```python
from build123d import *

# Parameters (mm, degrees)
F0_W     = 35
F0_H     = 80
F0_H_2   = 120
F2_DEPTH = 1
F4_DEPTH = 2000
F5_DEPTH = 640


# Not quite as in the source:
# - a feature names something its author has since deleted; it is built from what else it names


with BuildPart() as f2:
    # F0 (on Top) → F2 (new body)
    with BuildSketch(Plane.XY):
        Polygon((380, 360), (-380, 360), (-380, -360), (0, -360), (380, -360), align=None)
        with Locations((-260.5, -310)):
            Rectangle(F0_W, F0_H, mode=Mode.SUBTRACT)
        with Locations((260.5, -310)):
            Rectangle(F0_W, F0_H, mode=Mode.SUBTRACT)
        with Locations((-260.5, 250)):
            Rectangle(F0_W, F0_H_2, mode=Mode.SUBTRACT)
        with Locations((260.5, 250)):
            Rectangle(F0_W, F0_H_2, mode=Mode.SUBTRACT)
    extrude(amount=F2_DEPTH)

    # F0 (on Top) → F4 (join)
    with BuildSketch(Plane.XY):
        with Locations((-260.5, 250)):
            Rectangle(F0_W, F0_H_2)
        with Locations((-260.5, -310)):
            Rectangle(F0_W, F0_H)
        with Locations((260.5, -310)):
            Rectangle(F0_W, F0_H)
        with Locations((260.5, 250)):
            Rectangle(F0_W, F0_H_2)
    extrude(amount=F4_DEPTH)

    # F3 (on offset) → F5 (join)
    with BuildSketch(Plane.XZ.offset(350)):
        Polygon((-187.5, 29), (-187.5, 30), (-232.5, 30), (-242.5, 30), (-242.5, 40), (-242.5, 70), (-243.5, 70), (-243.5, 30), (-243.5, 29), align=None)
        Polygon((-242.5, 30), (-232.5, 30), (-242.5, 40), align=None)
        Polygon((242.5, 40), (232.5, 30), (242.5, 30), align=None)
        Polygon((232.5, 30), (187.5, 30), (187.5, 29), (243.5, 29), (243.5, 30), (243.5, 70), (242.5, 70), (242.5, 40), (242.5, 30), align=None)
    extrude(amount=-F5_DEPTH)


solid = f2.part
```
Can you work these out from the model? Positions are in its coordinate system, mm. A direction names the side the tool comes from. Round coordinates to 2 decimals unless told otherwise and drop trailing zeros. Loops run counter-clockwise (first coordinate to the right, second up) from the corner with the lowest first, then second, coordinate; pieces in that order, holes last. Notation, with made-up numbers: (30.25, 78.5) -> (65.25, 78.5) arc R35 ccw to (65.25, 117.5) -> close; hole circle Ø5 at (87, -16). An arc over 180 degrees is marked (long way). Answer in a Markdown table with one row per item.
Item 1: Suppose I cut it at B-B, the plane y = -238. List the corners of the cut face in (x, z) for me, plus the area to 3 significant figures.
Answer block:
| item | result |
|---|---|
| outline | (-380, 0) -> (380, 0) -> (380, 1) -> (-380, 1) -> close; (-243.5, 29) -> (-187.5, 29) -> (-187.5, 30) -> (-232.5, 30) -> (-242.5, 40) -> (-242.5, 70) -> (-243.5, 70) -> close; (187.5, 29) -> (243.5, 29) -> (243.5, 70) -> (242.5, 70) -> (242.5, 40) -> (232.5, 30) -> (187.5, 30) -> close |
| area | 1,050 mm² |
Item 2: Suppose I cut it at A-A, the plane z = 959. List the corners of the cut face in (x, y) for me.
Answer block:
| item | result |
|---|---|
| outline | (-278, -350) -> (-243, -350) -> (-243, -270) -> (-278, -270) -> close; (-278, 190) -> (-243, 190) -> (-243, 310) -> (-278, 310) -> close; (243, -350) -> (278, -350) -> (278, -270) -> (243, -270) -> close; (243, 190) -> (278, 190) -> (278, 310) -> (243, 310) -> close |
Item 3: Suppose I cut it at C-C, the plane x = -120.5. List the corners of the cut face in (y, z) for me.
Answer block:
| item | result |
|---|---|
| outline | (-360, 0) -> (360, 0) -> (360, 1) -> (-360, 1) -> close |
Item 4: If I drill on probe 1 along Y at (x, z) = (256, 755.5); probe 2 along X at (y, z) = (195, 1012.5); probe 3 along Z at (x, y) = (-198, 126), over which ranges is the centre line in solid material (lowest first)?
Answer block:
| item | result |
|---|---|
| probe 1 | -350 to -270, 190 to 310 |
| probe 2 | -278 to -243, 243 to 278 |
| probe 3 | 0 to 1, 29 to 30 |
Item 5: On a 3-axis mill with a long thin cutter (end or side, diameter ignored), from which of +Z, -Z, +X, -X, +Y, -Y can I reach the whole of each face in a straight line? I mean faces 1 (the flat face through (278, 249, 987)), 2 (the flat face through (-243, -311, 1021)), 3 (the flat face through (256, -350, 996)), 4 (the flat face through (260, -309, 2000)), 5 (the flat face through (-243.5, -43, 50)). Say none if no direction works.
Answer block:
| item | result |
|---|---|
| face 1 | +Z, +X, +Y, -Y |
| face 2 | +Z, +Y, -Y |
| face 3 | +Z, +X, -X, -Y |
| face 4 | +Z, +X, -X, +Y, -Y |
| face 5 | +Z, -X |
Item 6: Will these pins go through, and if not, where does the flat tip stop? P1, Ø10, axis at x = 239.5, y = -90.5, coming from the +Z side; P2, Ø24, axis at y = -316.5, z = 1509, coming from the +X side; P3, Ø9, axis at y = 85.5, z = 57, coming from the -X side.
Answer block:
| item | result |
|---|---|
| P1 | z = 70 |
| P2 | x = 278 |
| P3 | x = -243.5 |
Item 7: We'd pull the mould along Y, two halves only. Please class faces 6 (the flat face through (243.5, -43, 49)), 7 (the flat face through (-261, 190, 987)), 8 (the flat face through (-210, -34, 30)), 9 (the flat face through (260, 310, 987)): released by +Y, released by -Y, zero draft, split by the parting line, or undercut.
Answer block:
| item | result |
|---|---|
| face 6 | undercut |
| face 7 | undercut |
| face 8 | zero draft |
| face 9 | released by +Y |
